Design review of the part built by this model. Coordinates are the model's own, in mm. Face numbers are marked on the shaded views. Give positions to 0.01 mm unless a question says otherwise; leave off trailing zeros. Write each loop counter-clockwise with the first axis right and the second up, starting at its lowest first coordinate (ties: lowest second). Pieces come first, ordered by that corner, then holes. Notation, with made-up numbers: M -7.5,-30 L 19.5,-30 A30 ccw 19.5,4 Z; hole C 26,45 d8. An arc over 180 degrees is marked long. Write each question's results on one line, items separated by ' | '. Start each with the question number.
from build123d import *

# Parameters (mm, degrees)
F0_R     = 8
F1_DEPTH = 13


with BuildPart() as f1:
    # F0 (on Right) → F1 (new body)
    with BuildSketch(Plane.YZ):
        Polygon((12, 6.928203), (0, 13.856406), (-12, 6.928203), (-12, -6.928203), (0, -13.856406), (12, -6.928203), align=None)
        Circle(F0_R, mode=Mode.SUBTRACT)
    extrude(amount=F1_DEPTH)

    # F2 (on Front) → F3 (revolve, cut)
    with BuildSketch(Plane.XZ):
        Polygon((0, 24.532327), (0, 11), (3.625976, 24.532327), align=None)
        Polygon((9.374024, 24.532327), (13, 11), (13, 24.532327), align=None)
    revolve(axis=Axis((40.371262, 0, 0), (1, 0, 0)), mode=Mode.SUBTRACT)


solid = f1.part
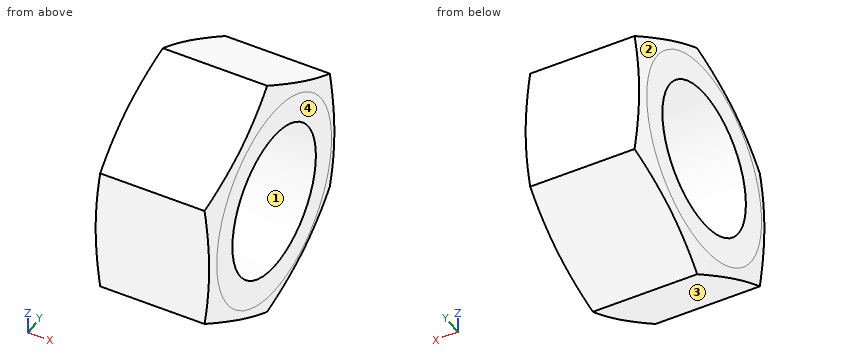
Q1. For pin 1 Ø6 at (x, y) = (7, 8.5) entering from -Z; pin 2 Ø1.5 at (x, y) = (6, -4.5) entering from -Z, all flat-tipped, find the tip position at first contact; note any pin that passes through.
Q2. We need section A-A on z = 0. Write out the cut boundary in (x, y).
Q3. The part is to be moulded in two halves that separate along Y. For the marked faces 1, 2, 3 and 4, say which applies: pulls with the +Y half, pulls with the -Y half, needs draft (parallel to the pull), parting line crosses it, or undercut.
Q4. We need section B-B on x = 3. Write out the cut boundary in (y, z).
Q5. Wall thickness on line 1 along Z through (x, y) = (8.25, 5.5); line 2 along Z through (x, y) = (5.5, -1); line 3 along Y through (x, z) = (1.25, 1.5): over which ranges is each line inside the solid? List them lowest first. Write a range as from..to.
Answer sheet:
1) pin 1: z = -10.68 | pin 2: z = -11.69
2) outline: M 0,-11 L 0.27,-12 L 12.73,-12 L 13,-11 L 13,-8 L 0,-8 Z; M 0,8 L 13,8 L 13,11 L 12.73,12 L 0.27,12 L 0,11 Z
3) face 1: undercut | face 2: parting line crosses it | face 3: pulls with the -Y half | face 4: needs draft
4) outline: M -12,-6.93 L 0,-13.86 L 12,-6.93 L 12,6.93 L 0,13.86 L -12,6.93 Z; hole C 0,0 d16
5) line 1: -10.68..-5.81, 5.81..10.68 | line 2: -13.28..-7.94, 7.94..13.28 | line 3: -12..-7.86, 7.86..12
